Could you check a few things on this drawing? It's one solid part, dimensions in mm from its lowest x, y, z. A direction names the side the tool comes from. Give positions to 0.01 mm unless a question says otherwise; leave off trailing zeros. Write each loop counter-clockwise with the first axis right and the second up, starting at its lowest first coordinate (ties: lowest second). Pieces come first, ordered by that corner, then holes. Notation, with made-up numbers: M 0,-35.5 L 52,-35.5 A14 ccw 52,-25.5 Z; hole C 13.5,1 d9. An arc over 180 degrees is marked long. Answer as CSV lines item,"result". Start each with the question number.
Q1. On a 3-axis mill with a long thin cutter (end or side, diameter ignored), from which of +Z, -Z, +X, -X, +Y, -Y can I reach the whole of each face in a straight line? I mean the marked faces 1 and 2. Say none if no direction works.
Q2. Suppose I cut it at C-C (z = 3.25). Write out the boundary of the cut face in (x, y).
Q3. If I drill on line 1 along Y through (x, z) = (16, 7.5); line 2 along X through (y, z) = (17, 7.25); line 3 along X through (y, z) = (6.5, 8.5), over which ranges is the centre line in solid material (lowest first)?
Q4. For pin 1 (5 mm diameter, centred on x = 16, y = 17, fed in from -Z); pin 2 (2 mm diameter, centred on y = 22.5, z = 15.5, fed in from -X); pin 3 (4 mm diameter, centred on x = 3.5, z = 6.5, fed in from +Y); pin 4 (5 mm diameter, centred on x = 22.5, z = 4, fed in from +Y), each with a flat end and sliding along its axis, tell me the tip position at first contact or that it passes through.
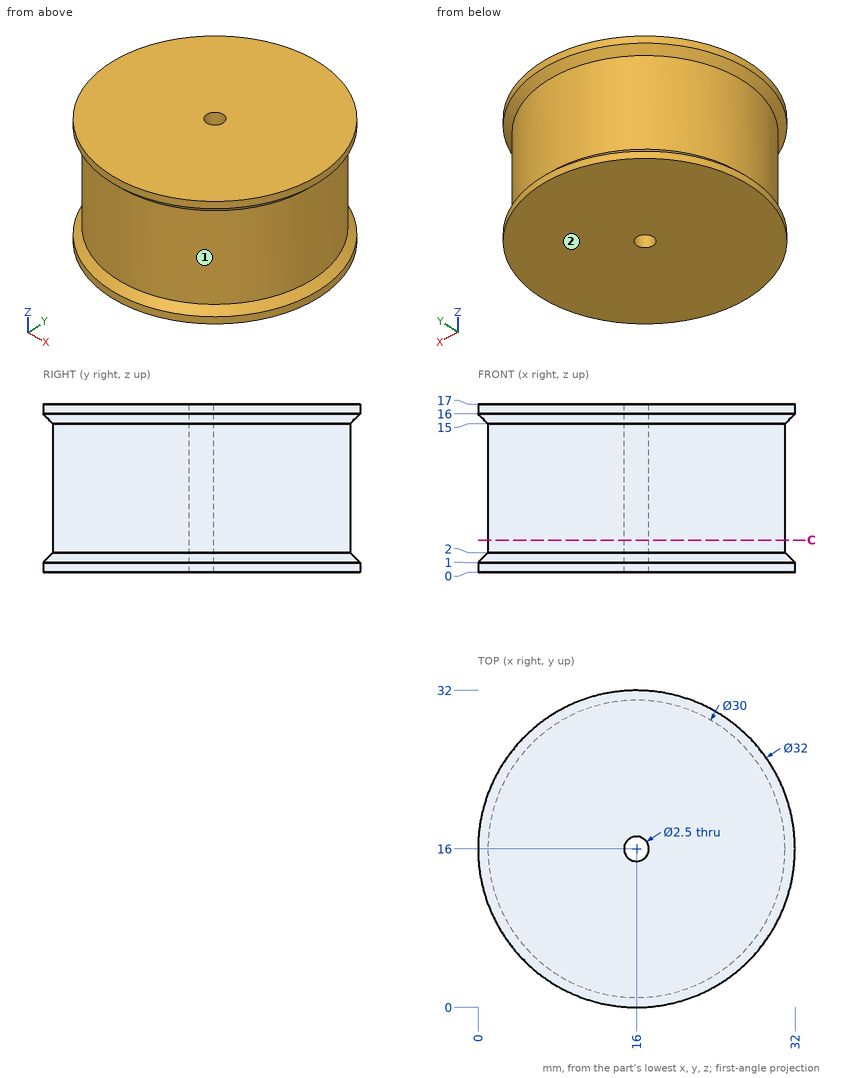
Resolved:
1,face 1,"none"
1,face 2,"-Z, +X, -X, +Y, -Y"
2,outline,"C 16,16 d30; hole C 16,16 d2.5"
3,line 1,"1 to 14.75, 17.25 to 31"
3,line 2,"1.03 to 15.25, 16.75 to 30.97"
3,line 3,"4.39 to 27.61"
4,pin 1,"z = 0"
4,pin 2,"x = 1.02"
4,pin 3,"y = 26.71"
4,pin 4,"y = 30.46"
